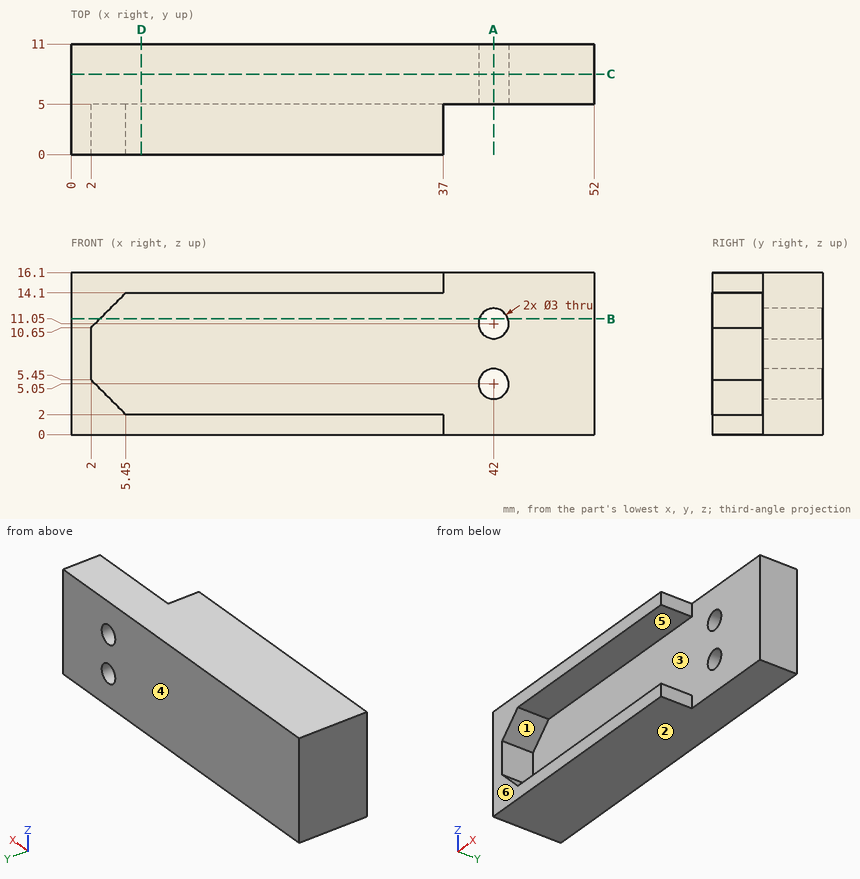
The drawing under review shows one solid part. Ordinate dimensions are in mm from its lowest x, y, z. A direction names the side the tool comes from. Give positions to 0.01 mm unless a question says otherwise; leave off trailing zeros. Order: outer loops, then holes, each group sorted by start corner. A loop starts at its lowest first (then second) coordinate and runs counter-clockwise, first axis right, second up. Notation, with made-up numbers: (77.5, 44.25) - (96.5, 44.25) arc R27 ccw to (96.5, 66.25) - close; hole circle Ø7 at (19.25, 60). An arc over 180 degrees is marked (long way). Answer as a JSON object with one key per item and string values. Group by question number.
Item 1: Take a section at D-D on x = 7. Give the boundary of the cut face in (y, z), and give its area (3 significant figures).
Item 2: Clearance check with flat-ended pins moving along their axes: pin 1 Ø4 at (y, z) = (1.5, 13.5) entering from +X; pin 2 Ø2.5 at (x, z) = (42, 11.05) entering from +Y (3 decimals); pin 3 Ø2 at (y, z) = (6.5, 7) entering from -X; pin 4 Ø4 at (x, z) = (42, 5.05) entering from -Y. State where each tip first meets the part, or that it passes through.
Item 3: Take a section at C-C on y = 8. Give the boundary of the cut face in (x, z).
Item 4: Draft analysis for pull direction Z (two halves, no side actions). For the marked faces 1, 2, 3 and 4, state which applies: pulls with the +Z half, pulls with the -Z half, needs draft (parallel to the pull), parting line crosses it, or undercut.
Item 5: Take a section at B-B on z = 11.5. Give the boundary of the cut face in (x, y), and give its area (3 significant figures).
Item 6: Wall thickness on line 1 along X through (y, z) = (9.3, 11.05); line 2 along Y through (x, z) = (38.5, 9.25); line 3 along X through (y, z) = (2.75, 9.5): over which ranges is each line inside the solid? List them lowest first.
Item 7: Take a section at A-A on x = 42. Give the boundary of the cut face in (y, z), and give its area (3 significant figures).
Item 8: Machinability: for the marked faces 5 and 6, which of the approach directions +Z, -Z, +X, -X, +Y, -Y give a long, thin tool a straight path to every point of the face, cutting with its end or side? Answer none if there is none.
Reported:
{
 "1": {"outline": "(0, 0) - (11, 0) - (11, 16.1) - (0, 16.1) - (0, 14.1) - (5, 14.1) - (5, 2) - (0, 2) - close", "area": "117 mm^2"},
 "2": {"pin 1": "x = 37", "pin 2": "through", "pin 3": "x = 0", "pin 4": "y = 5"},
 "3": {"outline": "(0, 0) - (52, 0) - (52, 16.1) - (0, 16.1) - close; hole circle Ø3 at (42, 5.05); hole circle Ø3 at (42, 11.05)"},
 "4": {"face 1": "undercut", "face 2": "pulls with the -Z half", "face 3": "undercut", "face 4": "needs draft"},
 "5": {"outline": "(0, 0) - (2.85, 0) - (2.85, 5) - (40.57, 5) - (40.57, 11) - (0, 11) - close; (43.43, 5) - (52, 5) - (52, 11) - (43.43, 11) - close", "area": "309 mm^2"},
 "6": {"line 1": "0 to 40.5, 43.5 to 52", "line 2": "5 to 11", "line 3": "0 to 2"},
 "7": {"outline": "(5, 0) - (11, 0) - (11, 3.55) - (5, 3.55) - close; (5, 6.55) - (11, 6.55) - (11, 9.55) - (5, 9.55) - close; (5, 12.55) - (11, 12.55) - (11, 16.1) - (5, 16.1) - close", "area": "60.6 mm^2"},
 "8": {"face 5": "+X, -Y", "face 6": "+Z, -Z, +X, -X, -Y"}
}
